Source: CAD feature listing. Evaluate the final solid. Frame: model axes, mm. A direction names the side the tool comes from. Give positions to 0.01 mm unless a question says otherwise; leave off trailing zeros. Order: outer loops, then holes, each group sorted by start corner. A loop starts at its lowest first (then second) coordinate and runs counter-clockwise, first axis right, second up. Notation, with made-up numbers: (49.5, 60.5) - (64.5, 60.5) arc R8 ccw to (64.5, 75.5) - close; hole circle Ø11 at (-30, 44.5). An arc over 180 degrees is marked (long way). Answer as CSV lines item,"result".
```python
from build123d import *

# Parameters (mm, degrees)
BOSS_EXTRUDE1_DEPTH     = 10
SKETCH2_W               = 83.569070853
SKETCH2_H               = 48.012038302
CUT_EXTRUDE1_DEPTH      = 12
CUT_EXTRUDE1_DEPTH_BACK = 12
BOSS_EXTRUDE2_DEPTH     = 5
BOSS_EXTRUDE3_DEPTH     = 5
SKETCH5_W               = 15.8
SKETCH5_H               = 47
CUT_EXTRUDE2_DEPTH      = 6.5


with BuildPart() as part:
    # Sketch1 → Boss-Extrude1 (new body)
    with BuildSketch(Plane(origin=(0, 0, 0), x_dir=(1, 0, 0), z_dir=(0, 1, 0))):
        with BuildLine():
            Line((10.2, -57.235021417), (10.2, 3.135021417))
            ThreePointArc((10.2, 3.135021417), (0, 3.88), (-10.2, 3.135021417))
            Line((-10.2, 3.135021417), (-10.2, -57.235021417))
            ThreePointArc((-10.2, -57.235021417), (0, -57.98), (10.2, -57.235021417))
        make_face()
    extrude(amount=BOSS_EXTRUDE1_DEPTH)

    # Sketch2 → Cut-Extrude1 (cut, two sides)
    with BuildSketch(Plane(origin=(0, 0, 0), x_dir=(0, 0, -1), z_dir=(1, 0, 0))) as cut_extrude1_sk:
        with Locations((-26.748669216, 4)):
            Rectangle(SKETCH2_W, SKETCH2_H)
        with BuildLine():
            Line((-57.98, 6.572226563), (-57.98, 3.5))
            Line((-57.98, 3.5), (-51.917822174, 0))
            Line((-51.917822174, 0), (-2.182177826, 0))
            Line((-2.182177826, 0), (3.88, 3.5))
            Line((3.88, 3.5), (3.88, 6.572226563))
            ThreePointArc((3.88, 6.572226563), (3.7441635, 6.914841427), (3.410460219, 7.071297876))
            ThreePointArc((3.410460219, 7.071297876), (-27.050000121, 8), (-57.51046046, 7.071297861))
            ThreePointArc((-57.51046046, 7.071297861), (-57.844163583, 6.914841339), (-57.98, 6.572226563))
        make_face(mode=Mode.SUBTRACT)
    extrude(amount=CUT_EXTRUDE1_DEPTH, mode=Mode.SUBTRACT)
    extrude(cut_extrude1_sk.sketch, amount=-CUT_EXTRUDE1_DEPTH_BACK, mode=Mode.SUBTRACT)

    # Sketch3 → Boss-Extrude2 (add)
    with BuildSketch(Plane(origin=(0, 0, 0), x_dir=(1, 0, 0), z_dir=(0, 1, 0))):
        with BuildLine():
            Line((-3.6, 0), (-3.6, -3.6))
            Line((-3.6, -3.6), (3.6, -3.6))
            Line((3.6, -3.6), (3.6, 0))
            ThreePointArc((3.6, 0), (0, 3.600000126), (-3.6, 0))
        make_face()
    extrude(amount=BOSS_EXTRUDE2_DEPTH)

    # Sketch4 → Boss-Extrude3 (add)
    with BuildSketch(Plane(origin=(0, 0, 0), x_dir=(1, 0, 0), z_dir=(0, 1, 0))):
        with BuildLine():
            Line((3.6, -54.1), (3.6, -50.5))
            Line((3.6, -50.5), (-3.6, -50.5))
            Line((-3.6, -50.5), (-3.6, -54.1))
            ThreePointArc((-3.6, -54.1), (0, -57.7), (3.6, -54.1))
        make_face()
    extrude(amount=BOSS_EXTRUDE3_DEPTH)

    # Sketch5 → Cut-Extrude2 (cut)
    with BuildSketch(Plane(origin=(0, 0, 0), x_dir=(1, 0, 0), z_dir=(0, 1, 0))):
        with Locations((0, -27.05)):
            Rectangle(SKETCH5_W, SKETCH5_H)
    extrude(amount=CUT_EXTRUDE2_DEPTH, mode=Mode.SUBTRACT)

    # Sketch6 → Cut-Revolve1 (revolve, cut)
    with BuildSketch(Plane(origin=(0, 0, 0), x_dir=(0, 0, -1), z_dir=(1, 0, 0))):
        Polygon((0, 0), (-1.5, 0), (-1.5, 2.4), (-1.35, 2.4), (-1.35, 3), (-1.7, 3.202072594), (-1.7, 4.7), (-3.2, 4.7), (-3.2, 8), (0, 8), align=None)
    revolve(axis=Axis((0, 8, 0), (0, -1, 0)), mode=Mode.SUBTRACT)

    # Sketch7 → Cut-Revolve2 (revolve, cut)
    with BuildSketch(Plane(origin=(0, 0, 0), x_dir=(0, 0, -1), z_dir=(1, 0, 0))):
        Polygon((-54.1, 0), (-55.6, 0), (-55.6, 2.4), (-55.45, 2.4), (-55.45, 3), (-55.8, 3.202072594), (-55.8, 4.7), (-57.3, 4.7), (-57.3, 8), (-54.1, 8), align=None)
    revolve(axis=Axis((0, 8, 54.1), (0, -1, 0)), mode=Mode.SUBTRACT)


solid = part.part
```
(1) Contact query for flat-ended pins moving along their axis: pin 1 (0.9 mm diameter, centred on x = 0, z = 0.5, fed in from -Y); pin 2 (5 mm diameter, centred on x = 0, z = 54.1, fed in from +Y); pin 3 (10 mm diameter, centred on x = 0, z = 0, fed in from +Y); pin 4 (1 mm diameter, centred on x = -4.5, y = 3.5, fed in from +Z). Output: stop coordinate, or through.
Completed:
pin 1,"through"
pin 2,"y = 4.7"
pin 3,"y = 7.51"
pin 4,"z = 57.87"
(2) Cut plane A-A (y = 5.25). Return loops of the section in (x, z), then the cut area to 3 significant figures.
Completed:
outline,"(-10.2, -3.14) arc R70.2 ccw to (10.2, -3.14) - (10.2, 57.24) arc R70.2 ccw to (-10.2, 57.24) - close; hole (-7.9, 3.55) - (7.9, 3.55) - (7.9, 50.55) - (-7.9, 50.55) - close; hole circle Ø6.4 at (0, 0); hole circle Ø6.4 at (0, 54.1)"
area,"445 mm²"
(3) Mould query, pull axis Z, two halves, no side actions, for faces 4 (the flat face through (0, 3, 50.55)), 5 (the flat face through (-3.6, 0.3, 53.5)), 6 (the flat face through (-2.41, 2.94, 57.01)). Classes: released by +Z, released by -Z, zero draft, split by the parting line, or undercut.
Completed:
face 4,"undercut"
face 5,"zero draft"
face 6,"released by +Z"
(4) Cut plane C-C (x = 6.75). Return loops of the section in (y, z), then the cut area to 3 significant figures.
Completed:
outline,"(0, 2.18) - (3.31, -3.55) - (7.04, -3.55) arc R0.5 ccw to (7.07, -3.41) arc R500 ccw to (7.07, 57.51) arc R0.5 ccw to (7.04, 57.65) - (3.31, 57.65) - (0, 51.92) - (0, 50.55) - (6.5, 50.55) - (6.5, 3.55) - (0, 3.55) - close"
area,"146 mm²"
(5) Cut plane D-D (x = 0). Give the number of separate pieces and of enclosed holes in the cut face, then the cut area to 3 significant figures.
Completed:
separate pieces,"3"
enclosed holes,"0"
area,"106 mm²"
(6) Access query for faces 1 (the flat face through (3.6, 0.3, 0.6)), 2 (the flat face through (0, 6.5, 27)), 3 (the cylindrical face through (-0.961, 6.085, 3.052)). Directions: +Z, -Z, +X, -X, +Y, -Y. A direction counts if a zero-diameter tool reaches every point of the face in a straight line with its end or side. Return the directions, or none.
Completed:
face 1,"-Z, +X, -Y"
face 2,"-Y"
face 3,"+Y"
(7) Ray query, line 1 (Z direction, x = 0, y = 2.9); line 2 (Z direction, x = 0, y = 3.7); line 3 (X direction, y = 4, z = 14.5). Return the intervals inside material, ascending. Write a range as from..to.
Completed:
line 1,"-3.6..-1.35, 1.35..3.55, 50.55..52.75, 55.45..57.7"
line 2,"-3.88..-1.7, 1.7..3.55, 50.55..52.4, 55.8..57.98"
line 3,"-10.2..-7.9, 7.9..10.2"
(8) Cut plane B-B (z = 8.5). Return loops of the section in (x, y), then the cut area to 3 significant figures.
Completed:
outline,"(-10.2, 0) - (-7.9, 0) - (-7.9, 6.5) - (7.9, 6.5) - (7.9, 0) - (10.2, 0) - (10.2, 7.66) - (-10.2, 7.66) - close"
area,"53.5 mm²"
